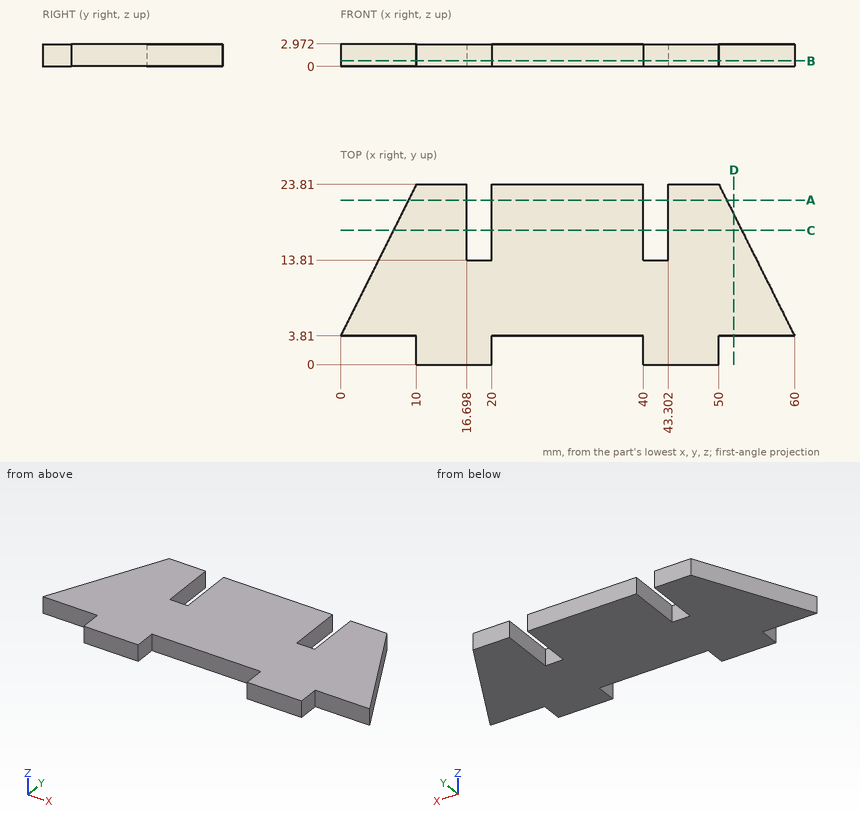
The figure shows three views and two pictorial views of one solid part (mm, origin at its lowest corner). Answer the questions. Round coordinates to 2 decimals unless told otherwise and drop trailing zeros. Write each loop counter-clockwise with the first axis right and the second up, starting at its lowest first coordinate (ties: lowest second). Pieces come first, ordered by that corner, then holes. Notation, with made-up numbers: (-12, -5) - (32, -5) arc R34 ccw to (32, 28) - close; hole circle Ø2 at (-35.75, 69). An arc over 180 degrees is marked (long way). Use one line per item in the form item = value. Start each with the question number.
Item 1: Flat-ended cylindrical pins translate along their axes: pin 1 Ø1.5 at (y, z) = (9, 2) entering from -X; pin 2 Ø1 at (x, z) = (52, 0.5) entering from +Y; pin 3 Ø0.9 at (y, z) = (2, 1) entering from -X. Find the tip coordinate at first contact, or state that the pin passes through.
Item 2: A cutting plane is placed at B-B (z = 0.75). Write down the section's boundary in (x, y), plus the area to 3 significant figures.
Item 3: A cutting plane is placed at A-A (y = 21.75). Write down the section's boundary in (x, z).
Item 4: A cutting plane is placed at C-C (y = 17.75). Write down the section's boundary in (x, z), plus the area to 3 significant figures.
Item 5: A cutting plane is placed at D-D (x = 52). Write down the section's boundary in (y, z).
Item 6: Find the intervals of material crossed by line 1 (X direction, y = 1.5, z = 2.6); line 2 (X direction, y = 16.5, z = 0.2) (1 decimal); line 3 (X direction, y = 14.5, z = 0.7) (1 decimal), in increasing order. Write a range as [from, to].
The answers:
q1.pin_1 = 2.22
q1.pin_2 = 20.81
q1.pin_3 = 10
q2.outline = (0, 3.81) - (10, 3.81) - (10, 0) - (20, 0) - (20, 3.81) - (40, 3.81) - (40, 0) - (50, 0) - (50, 3.81) - (60, 3.81) - (50, 23.81) - (43.3, 23.81) - (43.3, 13.81) - (40, 13.81) - (40, 23.81) - (20, 23.81) - (20, 13.81) - (16.7, 13.81) - (16.7, 23.81) - (10, 23.81) - close
q2.area = 1,010 mm^2
q3.outline = (8.97, 0) - (16.7, 0) - (16.7, 2.97) - (8.97, 2.97) - close; (20, 0) - (40, 0) - (40, 2.97) - (20, 2.97) - close; (43.3, 0) - (51.03, 0) - (51.03, 2.97) - (43.3, 2.97) - close
q4.outline = (6.97, 0) - (16.7, 0) - (16.7, 2.97) - (6.97, 2.97) - close; (20, 0) - (40, 0) - (40, 2.97) - (20, 2.97) - close; (43.3, 0) - (53.03, 0) - (53.03, 2.97) - (43.3, 2.97) - close
q4.area = 117 mm^2
q5.outline = (3.81, 0) - (19.81, 0) - (19.81, 2.97) - (3.81, 2.97) - close
q6.line_1 = [10, 20], [40, 50]
q6.line_2 = [6.3, 16.7], [20, 40], [43.3, 53.7]
q6.line_3 = [5.3, 16.7], [20, 40], [43.3, 54.7]
